Verification items for the finished model (mm, model axes). A direction names the side the tool comes from. Round coordinates to 2 decimals unless told otherwise and drop trailing zeros. Order: outer loops, then holes, each group sorted by start corner. A loop starts at its lowest first (then second) coordinate and runs counter-clockwise, first axis right, second up. Notation, with made-up numbers: (13.5, -16.75) -> (53.5, -16.75) arc R16 cw to (53.5, 1.25) -> close; hole circle Ø10 at (48.5, 41). An arc over 180 degrees is marked (long way). Write item = value, one per line. Start each with the question number.
Autodesk Inventor part; units mm, degrees
ref_plane "Arbeitsebene1" through (-75, 27.1, 0) normal (0, 0, 1) x (0, 1, 0)
ref_plane "Arbeitsebene2" through (0, 99.4, -2.4) normal (-1, 0, 0) x (0, 0, 1)
ref_plane "YZ Plane" through (0, 0, 0) normal (1, 0, 0) x (0, 1, 0)
ref_plane "Arbeitsebene1" through (-75, 27.1, 0) normal (0, 0, 1) x (0, 1, 0)
sketch "center1" plane through (-75, 27.1, 0) normal (0, 0, 1) x (0, 1, 0)
  line L0 (-173.891, -75) -> (168.1592, -75)
  line L1 (0, 239.86) -> (0, -220.81)
  point P0 (-27.1, -75)
ref_plane "Arbeitsebene2" through (0, 99.4, -2.4) normal (-1, 0, 0) x (0, 0, 1)
sketch "center2" plane through (0, 99.4, -2.4) normal (-1, 0, 0) x (0, 0, 1)
  line L0 (184.8129, -72.3) -> (-258.9785, -72.3)
  point P0 (2.4, -99.4)
sketch "Hallsens" plane through (0, 0, 0) normal (0, 1, 0) x (-1, 0, 0)
  line L0 (406.994, 0) -> (-237.944, 0) construction
  line L1 (0, -350.1368) -> (0, 271.1712) construction
  line L2 (-5, 0) -> (5, 0) construction
  line L3 (5, 0) -> (5, -20) construction
  line L4 (5, -20) -> (-5, -20) construction
  line L5 (-5, -20) -> (-5, 0) construction
  line L6 (-4, -1) -> (-6, -1)
  line L7 (-6, -1) -> (-6, 1)
  line L8 (-6, 1) -> (-4, 1)
  line L9 (-4, 1) -> (-4, -1)
  line L10 (-4, -1) -> (-6, 1) construction
  line L11 (-6, -1) -> (-4, 1) construction
  line L12 (4, -1) -> (6, -1)
  line L13 (6, -1) -> (6, 1)
  line L14 (6, 1) -> (4, 1)
  line L15 (4, 1) -> (4, -1)
  line L16 (4, -1) -> (6, 1) construction
  line L17 (6, -1) -> (4, 1) construction
  line L18 (4, -21) -> (6, -21)
  line L19 (6, -21) -> (6, -19)
  line L20 (6, -19) -> (4, -19)
  line L21 (4, -19) -> (4, -21)
  line L22 (4, -21) -> (6, -19) construction
  line L23 (6, -21) -> (4, -19) construction
  line L24 (-6, -21) -> (-4, -21)
  line L25 (-4, -21) -> (-4, -19)
  line L26 (-4, -19) -> (-6, -19)
  line L27 (-6, -19) -> (-6, -21)
  line L28 (-6, -21) -> (-4, -19) construction
  line L29 (-4, -21) -> (-6, -19) construction
  line L30 (-9, 10) -> (9, 10) construction
  line L31 (9, 10) -> (9, -40) construction
  line L32 (9, -40) -> (-9, -40) construction
  line L33 (-9, -40) -> (-9, 10) construction
  circle A0 centre (0, 10) radius 1.6
  circle A1 centre (9, -40) radius 1.6
  circle A2 centre (-9, -40) radius 1.6
  dimension "d126" = 10
  dimension "d127" = 20
  dimension "d128" = 5
  dimension "d129" = 2
  dimension "d130" = 4
  dimension "d131" = 4
  dimension "d132" = 10
  dimension "d133" = 20
  dimension "d134" = 3.2
sketch "Groundplane" plane through (0, 0, 0) normal (0, 1, 0) x (-1, 0, 0)
  line L0 (45, 45) -> (-45, 45) construction
  line L1 (-45, 45) -> (-45, -45) construction
  line L2 (-45, -45) -> (45, -45) construction
  line L3 (45, -45) -> (45, 45) construction
  line L4 (1, 45) -> (-1, 45) construction
  line L5 (-1, 45) -> (-1, 40) construction
  line L6 (-1, 40) -> (1, 40) construction
  line L7 (1, 40) -> (1, 45) construction
  arc A0 (-1, 40) -> (1, 40) centre (0, 40) ccw construction
  line L8 (1, -45) -> (-1, -45) construction
  line L9 (-1, -45) -> (-1, -40) construction
  line L10 (-1, -40) -> (1, -40) construction
  line L11 (1, -40) -> (1, -45) construction
  arc A1 (1, -40) -> (-1, -40) centre (0, -40) ccw construction
  point P0 (0, 0)
  dimension "d5" = 2
  dimension "d6" = 5
  dimension "d7" = 2
  dimension "d8" = 5
  dimension "d9" = 90
  dimension "d89" = 45
  dimension "d90" = 45
sketch "Montagepunkte" plane through (0, 0, 0) normal (0, 1, 0) x (-1, 0, 0)
  circle A0 centre (0, 10) radius 1.6
  circle A1 centre (9, -40) radius 1.6
  circle A2 centre (-9, -40) radius 1.6
  arc A3 (1, -40) -> (-1, -40) centre (0, -40) ccw construction
  arc A4 (-1, 40) -> (1, 40) centre (0, 40) ccw construction
  circle A5 centre (0, 40) radius 1
  circle A6 centre (0, -40) radius 1
  line L0 (-9, -40) -> (9, -40) construction
  line L1 (9, -40) -> (9, -20) construction
  line L2 (9, -20) -> (-9, -20) construction
  line L3 (-9, -20) -> (-9, -40) construction
  line L4 (0, 10) -> (0, 30) construction
  circle A7 centre (9, -20) radius 1.6
  circle A8 centre (-9, -20) radius 1.6
  circle A9 centre (0, 30) radius 1.6
  dimension "d135" = 2
  dimension "d136" = 20
  dimension "d137" = 20
  dimension "d138" = 3.2
sketch "Skizze5" plane through (0, 0, 0) normal (0, 1, 0) x (-1, 0, 0)
  line L0 (45, 45) -> (-45, 45)
  line L1 (-45, 45) -> (-45, -45)
  line L2 (-45, -45) -> (45, -45)
  line L3 (45, -45) -> (45, 45)
  circle A0 centre (0, 40) radius 1
  circle A1 centre (0, -40) radius 1
extrude "Extrusion2" add sketch "Skizze5" along normal blind 5
sketch "Skizze6" plane through (0, 5, 0) normal (0, 1, 0) x (1, 0, 0)
  line L0 (-5, -5) -> (5, -5)
  line L1 (5, -5) -> (5, -35)
  line L2 (5, -35) -> (-5, -35)
  line L3 (-5, -35) -> (-5, -5)
  line L4 (-14, 45) -> (14, 45)
  line L5 (14, 45) -> (14, 15)
  line L6 (14, 15) -> (-14, 15)
  line L7 (-14, 15) -> (-14, 45)
  circle A0 centre (0, -40) radius 1
  circle A1 centre (0, -40) radius 1
  circle A2 centre (0, -30) radius 1.6
  circle A3 centre (0, -10) radius 1.6
  circle A4 centre (-9, 20) radius 1.6
  circle A5 centre (9, 20) radius 1.6
  circle A6 centre (9, 40) radius 1.6
  circle A7 centre (-9, 40) radius 1.6
  circle A8 centre (0, 40) radius 1
  point P0 (0, 0)
  dimension "d139" = 5
  dimension "d140" = 5
  dimension "d141" = 5
  dimension "d142" = 5
  dimension "d143" = 5
  dimension "d144" = 5
  dimension "d145" = 5
  dimension "d146" = 5
extrude "Extrusion3" add sketch "Skizze6" along normal blind 3 contours L0 L1 L2 L3 | L4 L5 L6 L7
chamfer "Fase1" distance 1 distance2 3 4 edges at (7.4, 8, -20) (-10.6, 8, -20) (-10.6, 8, -40) (7.4, 8, -40) measured on face at (0.0402, 8, -27.0431)
chamfer "Fase2" distance 1 distance2 3 2 edges at (-1.6, 8, 30) (-1.6, 8, 10) measured on face at (3.8056, 8, 16.9145)
sketch "Skizze8" plane through (0, 8, 0) normal (0, 1, 0) x (1, 0, 0)
  circle A0 centre (0, 40) radius 3
  circle A1 centre (0, 40) radius 1
  circle A2 centre (0, 40) radius 1
  circle A3 centre (0, 40) radius 1
  point P0 (0, 0)
  dimension "d99" = 6
extrude "Extrusion5" cut sketch "Skizze8" against normal up to surface (3 mm away) contours A0 | A1
sketch "Skizze9" plane through (0, 5, 0) normal (0, 1, 0) x (1, 0, 0)
  line L0 (15, 40) -> (40, 40)
  line L1 (40, 40) -> (40, -40)
  line L2 (40, -40) -> (15, -40)
  line L3 (15, -40) -> (15, 40)
  line L4 (15, 40) -> (15, -40) construction
  line L5 (31, 28) -> (31, 18)
  line L6 (31, 25) -> (15, 25)
  line L7 (31, 21) -> (15, 21)
  line L8 (15, 21) -> (15, 25)
  line L9 (31, 28) -> (41, 24.4341)
  line L10 (41, 24.4341) -> (41, 21.5659)
  line L11 (41, 21.5659) -> (31, 18)
  line L12 (-40, 10) -> (10, 10)
  line L13 (10, 10) -> (10, 0)
  line L14 (10, 0) -> (-40, 0)
  line L15 (-40, 0) -> (-40, 10)
  line L16 (-40, -5) -> (-10, -5)
  line L17 (-10, -5) -> (-10, -40)
  line L18 (-10, -40) -> (-40, -40)
  line L19 (-40, -40) -> (-40, -5)
  line L20 (-5, -5) -> (-5, -35)
  line L21 (-14, 15) -> (14, 15)
  line L22 (5, -5) -> (-5, -5)
  line L23 (-45, -45) -> (45, -45) construction
  line L24 (45, -45) -> (45, 45) construction
  line L25 (45, 45) -> (14, 45) construction
  line L26 (-14, 45) -> (-45, 45) construction
  line L27 (-45, 45) -> (-45, -45) construction
  point P0 (0, 0)
  point P1 (9, 45)
  point P2 (40, 23)
  point P3 (31, 23)
  point P4 (41, 23)
  point P5 (40, 21.2093)
  point P6 (40, 24.7907)
  point P7 (-40, -22.5)
  dimension "d106" = 25
  dimension "d107" = 0
  dimension "d108" = 3
  dimension "d109" = 3
  dimension "d110" = 4
  dimension "d111" = 9
  dimension "d112" = 15
  dimension "d115" = 1
  dimension "d118" = 5
  dimension "d119" = 5
  dimension "d123" = 5
  dimension "d124" = 5
  dimension "d125" = 5
  dimension "d147" = 5
  dimension "d148" = 5
  dimension "d149" = 5
  dimension "d150" = 5
  dimension "d151" = 5
  dimension "d152" = 5
extrude "Extrusion6" cut sketch "Skizze9" against normal through all contours L0 L1 L9 L5 L6 L3 | L7 L5 L11 L1 L2 L3 | L12 L13 L14 L15 | L16 L17 L18 L19
sketch "Skizze10" plane through (0, 5, 0) normal (0, 1, 0) x (1, 0, 0)
  line L0 (15, -40) -> (15, 21) construction
  line L1 (42, 2.9607) -> (26.2682, -6.3602)
  line L2 (26.2682, -6.3602) -> (15, -6.3602)
  line L3 (15, -6.3602) -> (15, -13.143)
  line L4 (15, -13.143) -> (25.94, -13.143)
  line L5 (25.94, -13.143) -> (42, -22.6171)
  line L6 (42, -22.6171) -> (42, -14.8934)
  line L7 (42, -14.8934) -> (32.3728, -9.6203)
  line L8 (32.3728, -9.6203) -> (42, -4.5223)
  line L9 (42, -4.5223) -> (42, 2.9607)
  point P0 (0, 0)
extrude "Extrusion7" add sketch "Skizze10" against normal up to surface (5 mm away)
properties part number "HallSensor_Halterung"
(1) Cross-section at C-C (z = 25.5). Enter the section's corners in (x, y), and give its area (3 significant figures).
(2) Cross-section at D-D (y = 1.75). Give the number of separate pieces and of enclosed holes in the cut face, and give its area (3 significant figures).
(3) Cross-section at B-B (x = 18). Enter the section's corners in (y, z).
(4) Set-up check for faces 1 (the flat face through (0, 6, 5)), 2 (the flat face through (36.24, 2.54, 11.74)), 3 (the flat face through (-9, 5, -40)), 4 (the flat face through (-5, 6, 20)): record each of +Z, -Z, +X, -X, +Y, -Y from which the full face is reachable in a straight line by a thin tool's end or side.
(5) Cross-section at A-A (z = -35). Enter the section's corners in (x, y).
(6) Draft check along Z on faces 5 (the flat face through (-45, 2, -1)), 6 (the flat face through (-40, 3, 23)). Enter one of: +Z half, -Z half, draft (parallel to the pull), parting line (faces both ways), or undercut.
(7) Depth check by flat-ended pin: pin 1 (1.6 mm diameter, centred on x = 8.5, z = -39.5, fed in from +Y); pin 2 (0.9 mm diameter, centred on y = 6, z = 22, fed in from -X); pin 3 (1.5 mm diameter, centred on x = 7, y = 6.5, fed in from +Z). Enter the tip coordinate at first touch or a pass-through.
(8) Scan lines: line 1 along Z through (x, y) = (-12, 3.5); line 2 along Z through (x, y) = (9, 5.05); line 3 along Z through (x, y) = (0, 3.15). Record each from-to range of solid material in increasing order. Write a range as from..to.
Outcome:
q1.outline = (-45, 0) -> (-40, 0) -> (-40, 5) -> (-45, 5) -> close; (-10, 0) -> (15, 0) -> (15, 5) -> (5, 5) -> (5, 8) -> (-5, 8) -> (-5, 5) -> (-10, 5) -> close; (40, 0) -> (45, 0) -> (45, 5) -> (40, 5) -> close
q1.area = 205 mm^2
q2.separate_pieces = 1
q2.enclosed_holes = 8
q2.area = 4,920 mm^2
q3.outline = (0, -45) -> (5, -45) -> (5, -40) -> (0, -40) -> close; (0, -25) -> (5, -25) -> (5, -21) -> (0, -21) -> close; (0, 6.36) -> (5, 6.36) -> (5, 13.14) -> (0, 13.14) -> close; (0, 40) -> (5, 40) -> (5, 45) -> (0, 45) -> close
q4.face_1 = +X, -X, +Y
q4.face_2 = +Y, -Y
q4.face_3 = +Y
q4.face_4 = +Z, -X, +Y
q5.outline = (-45, 0) -> (15, 0) -> (15, 5) -> (14, 5) -> (14, 8) -> (-14, 8) -> (-14, 5) -> (-45, 5) -> close; (40, 0) -> (45, 0) -> (45, 5) -> (40, 5) -> close
q6.face_5 = draft
q6.face_6 = undercut
q7.pin_1 = 5
q7.pin_2 = -5
q7.pin_3 = -15
q8.line_1 = -45..-10, 0..5, 40..45
q8.line_2 = -45..-41.62, -38.38..-21.62, -18.38..-15
q8.line_3 = -45..-41, -39..-10, 0..39, 41..45
